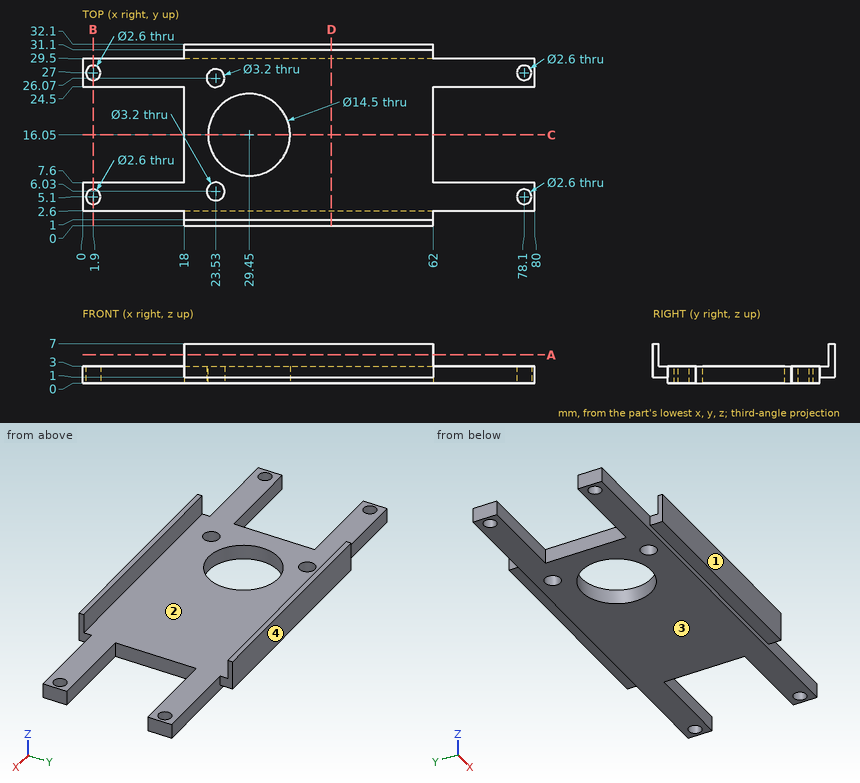
Print and shaded views of the part. All mm, measured from the part's lowest x, y and z. Coordinates: 2 decimals unless noted, no trailing zeros. Loops run counter-clockwise (first coordinate to the right, second up) from the corner with the lowest first, then second, coordinate; pieces in that order, holes last. Notation, with made-up numbers: (68.25, -22.75) - (97.25, -22.75) arc R12 ccw to (97.25, -0.75) - close; hole circle Ø8 at (58.25, -9). An arc over 180 degrees is marked (long way). Write item = value, one per line. Start each with the question number.
Item 1: Pull direction Y, two halves, no side cores. Call the marked faces 1, 2, 3 and 4: +Y half, -Y half, draft (parallel to the pull), parting line (faces both ways), or undercut.
Item 2: Saw through at C-C, the plane y = 16.05. List the corners of the cut face in (x, z).
Item 3: Saw through at A-A, the plane z = 5. List the corners of the cut face in (x, y), then the cut area to 3 significant figures.
Item 4: Saw through at B-B, the plane x = 1.9. List the corners of the cut face in (y, z), then the cut area to 3 significant figures.
Item 5: Saw through at D-D, the plane x = 44. List the corners of the cut face in (y, z).
Item 6: Wall check: probe 1 along Y at (x, z) = (78.1, 1.3); probe 2 along Y at (x, z) = (69.5, 2.25); probe 3 along Y at (x, z) = (25, 4.5). Give the ranges that are in metal, low to high. Write a range as [from, to].
Item 7: Drop flat-ended pins along their axis: pin 1 Ø3 at (x, y) = (29.5, 3.5) entering from +Z; pin 2 Ø0.9 at (x, z) = (67, 2) entering from +Y; pin 3 Ø2.5 at (x, z) = (67, 1) entering from -Y; pin 4 Ø1.6 at (x, y) = (78.1, 27) entering from -Z. Give the stop position or say it passes through.
Answers:
q1.face_1 = -Y half
q1.face_2 = undercut
q1.face_3 = draft
q1.face_4 = +Y half
q2.outline = (18, 0) - (22.2, 0) - (22.2, 3) - (18, 3) - close; (36.7, 0) - (62, 0) - (62, 3) - (36.7, 3) - close
q3.outline = (18, 0) - (62, 0) - (62, 1) - (18, 1) - close; (18, 31.1) - (62, 31.1) - (62, 32.1) - (18, 32.1) - close
q3.area = 88.0 mm2
q4.outline = (2.6, 0) - (3.8, 0) - (3.8, 3) - (2.6, 3) - close; (6.4, 0) - (7.6, 0) - (7.6, 3) - (6.4, 3) - close; (24.5, 0) - (25.7, 0) - (25.7, 3) - (24.5, 3) - close; (28.3, 0) - (29.5, 0) - (29.5, 3) - (28.3, 3) - close
q4.area = 14.4 mm2
q5.outline = (0, 1) - (2.6, 1) - (2.6, 0) - (29.5, 0) - (29.5, 1) - (32.1, 1) - (32.1, 7) - (31.1, 7) - (31.1, 3) - (1, 3) - (1, 7) - (0, 7) - close
q6.probe_1 = [2.6, 3.8], [6.4, 7.6], [24.5, 25.7], [28.3, 29.5]
q6.probe_2 = [2.6, 7.6], [24.5, 29.5]
q6.probe_3 = [0, 1], [31.1, 32.1]
q7.pin_1 = 3
q7.pin_2 = 29.5
q7.pin_3 = 2.6
q7.pin_4 = through
